from build123d import *

# Parameters (mm, degrees)
SKETCH1_W           = 131.01574
SKETCH1_H           = 63.5
BOSS_EXTRUDE1_DEPTH = 1.21412
SKETCH2_W           = 63.5
SKETCH2_H           = 12.7
CUT_EXTRUDE1_DEPTH  = 2.21412


with BuildPart() as part:
    # Sketch1 → Boss-Extrude1 (new body)
    with BuildSketch(Plane(origin=(0, 0, 0), x_dir=(1, 0, 0), z_dir=(0, 1, 0))):
        Rectangle(SKETCH1_W, SKETCH1_H)
    extrude(amount=BOSS_EXTRUDE1_DEPTH)

    # Sketch2 → Cut-Extrude1 (cut, through all)
    with BuildSketch(Plane(origin=(0, 1.21412, 0), x_dir=(1, 0, 0), z_dir=(0, 1, 0))):
        with Locations((0, 9.525)):
            Rectangle(SKETCH2_W, SKETCH2_H)
    extrude(amount=-CUT_EXTRUDE1_DEPTH, mode=Mode.SUBTRACT)


solid = part.part
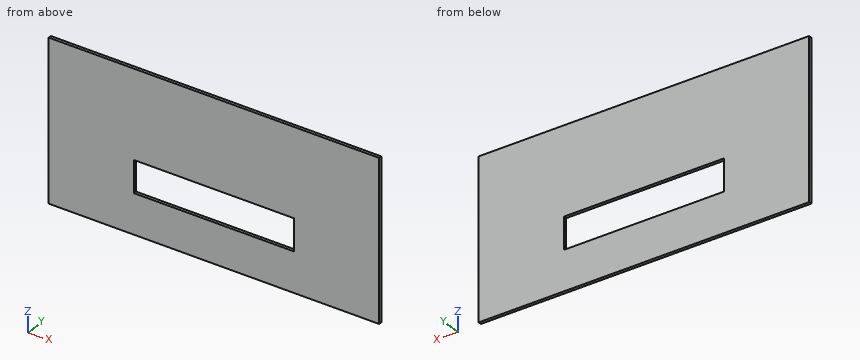
The listing builds one solid part. Answer for the finished solid, in the listing's coordinates (mm). Give positions to 0.01 mm unless a question says otherwise; leave off trailing zeros. Loops run counter-clockwise (first coordinate to the right, second up) from the corner with the lowest first, then second, coordinate; pieces in that order, holes last. Notation, with made-up numbers: (-11, 33.5) - (-2, 33.5) arc R28 cw to (-2, 52.5) - close; hole circle Ø3 at (54.5, 15.25). An arc over 180 degrees is marked (long way). Write each question's results on one line, items separated by ' | '.
1. Find section C-C, the plane y = 0.5. Write down the section's boundary in (x, z) (3 decimals).
Resolved:
outline: (-65.508, -31.75) - (65.508, -31.75) - (65.508, 31.75) - (-65.508, 31.75) - close; hole (-31.75, -15.875) - (31.75, -15.875) - (31.75, -3.175) - (-31.75, -3.175) - close
2. Consider probe 1 along Z at (x, y) = (11.5, 1.05) (3 decimals); probe 2 along X at (y, z) = (0.85, -15.5). Determine where each line is inside the solid, lowest interval first. Write a range as from..to.
Resolved:
probe 1: z = -31.75..-15.875, -3.175..31.75 | probe 2: x = -65.51..-31.75, 31.75..65.51
3. Find section B-B, the plane z = -13.5. Write down the section's boundary in (x, y), then the cut area to 3 significant figures.
Resolved:
outline: (-65.51, 0) - (-31.75, 0) - (-31.75, 1.21) - (-65.51, 1.21) - close; (31.75, 0) - (65.51, 0) - (65.51, 1.21) - (31.75, 1.21) - close | area: 82.0 mm^2
4. Find section A-A, the plane x = 20. Write down the section's boundary in (y, z) (3 decimals).
Resolved:
outline: (0, -31.75) - (1.214, -31.75) - (1.214, -15.875) - (0, -15.875) - close; (0, -3.175) - (1.214, -3.175) - (1.214, 31.75) - (0, 31.75) - close
